Design review of the part shown in the three views and the two pictorial views. Dimensions are in mm from the part's minimum x, y and z. Coordinates: 2 decimals unless noted, no trailing zeros. Write each loop counter-clockwise with the first axis right and the second up, starting at its lowest first coordinate (ties: lowest second). Pieces come first, ordered by that corner, then holes.
Q1. For L1, parallel to Y at x = 12, z = 3.25; L2, parallel to Y at x = 7.75, z = 3.5 (1 decimal); L3, parallel to X at y = 8.5, z = 4.5 (1 decimal), list the stretches that pass through material, from the lowest coordinate up.
Q2. The part is to be moulded in two halves that separate along Y. For the marked faces 1, 2, 3 and 4, say which applies: released by +Y, released by -Y, zero draft, split by the parting line, or undercut.
Q3. For pin 1 Ø4 at (x, y) = (18.5, 11.5) entering from -Z; pin 2 Ø1 at (y, z) = (15.5, 6) entering from +X, all flat-tipped, find the tip position at first contact; note any pin that passes through.
Q4. Take a section at A-A, the plane z = 4.5. Write out the cut boundary in (x, y) (1 decimal), plus the area to 3 significant figures.
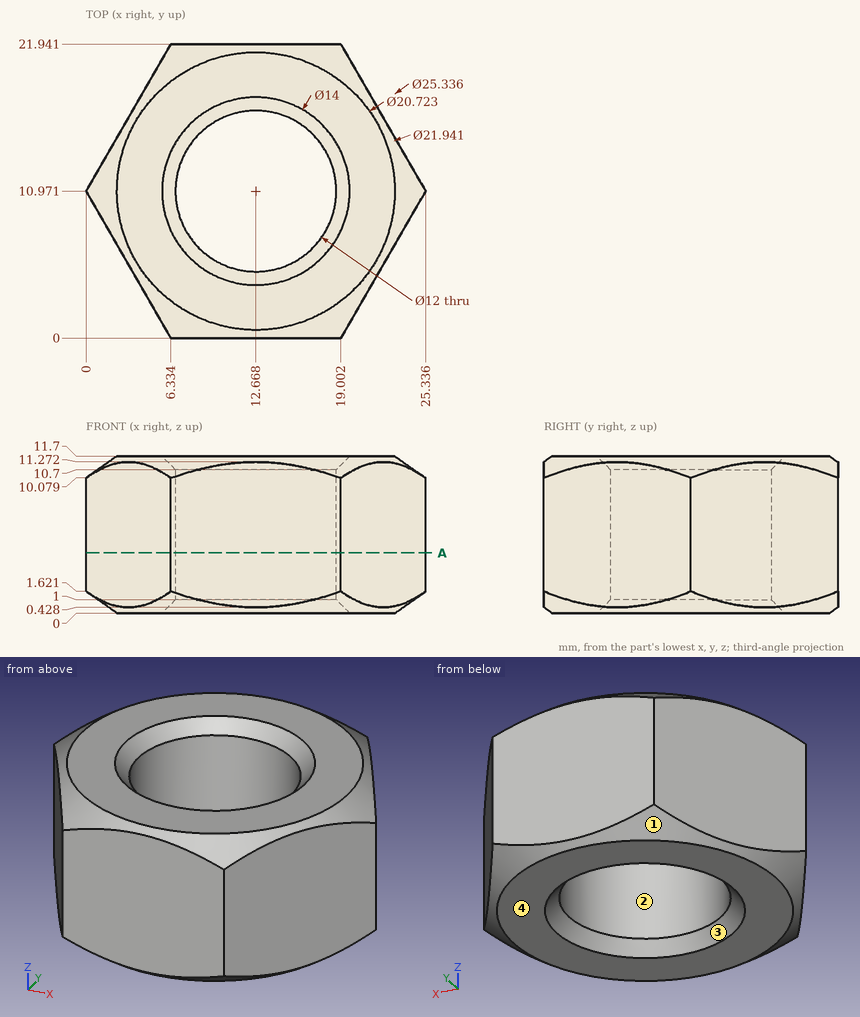
Responses:
1. L1: y = 0 to 5.01, 16.93 to 21.94
1. L2: y = 0 to 7.5, 14.4 to 21.9
1. L3: x = 1.4 to 7.2, 18.1 to 23.9
2. face 1: split by the parting line
2. face 2: undercut
2. face 3: undercut
2. face 4: zero draft
3. pin 1: stops at z = 0
3. pin 2: stops at x = 23.01
4. outline: (0, 11) - (6.3, 0) - (19, 0) - (25.3, 11) - (19, 21.9) - (6.3, 21.9) - close; hole circle Ø12 at (12.7, 11)
4. area: 304 mm2
